Input: part model. Units: mm. Frame: model coordinates. Face numbers are marked on the shaded views. Round coordinates to 2 decimals unless told otherwise and drop trailing zeros. Loops run counter-clockwise (first coordinate to the right, second up) from the corner with the lowest first, then second, coordinate; pieces in that order, holes last.
(1) Cut plane D-D, the plane x = -29. Output: boundary loops of the cut face in (y, z) (3 decimals).
(2) Cut plane B-B, the plane z = 3.5. Output: boundary loops of the cut face in (x, y) (3 decimals).
(3) Line query: line 1 (X direction, y = 67.5, z = 5) (3 decimals); line 2 (Z direction, x = -6.5, y = 2); line 3 (X direction, y = 22.5, z = 1). Output: solid intervals per line, ascending.
(4) Cut plane A-A, the plane y = 81. Output: boundary loops of the cut face in (x, z) (1 decimal).
(5) Draft query along X for the marked faces 1 and 2. Return one class per face: released by +X, released by -X, zero draft, split by the parting line, or undercut.
(6) Cut plane C-C, the plane x = 0. Output: boundary loops of the cut face in (y, z) (1 decimal).
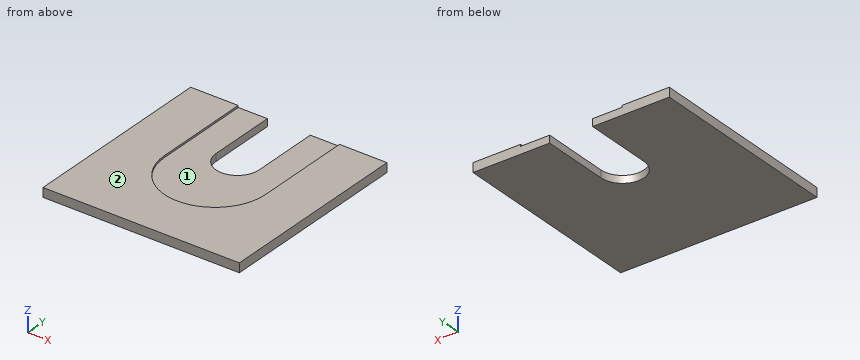
from build123d import *

# Parameters (mm, degrees)
F1_DEPTH = 9.525
F2_DEPTH = 7.62


# Not quite as in the source:
# - a feature names something its author has since deleted; it is built from what else it names


with BuildPart() as f1:
    # F0 (on Top) → F1 (new body)
    with BuildSketch(Plane.XY):
        with BuildLine():
            Line((-101.6, 101.6), (-101.6, -101.6))
            Line((-101.6, -101.6), (101.6, -101.6))
            Line((101.6, -101.6), (101.6, 101.6))
            Line((101.6, 101.6), (52.3875, 101.6))
            Line((52.3875, 101.6), (52.3875, 0))
            ThreePointArc((52.3875, 0), (0, -52.3875), (-52.3875, 0))
            Line((-52.3875, 0), (-52.3875, 101.6))
            Line((-52.3875, 101.6), (-101.6, 101.6))
        make_face()
    extrude(amount=F1_DEPTH)

    # F0 (on Top) → F2 (join)
    with BuildSketch(Plane.XY):
        with BuildLine():
            Line((-22.225, 101.6), (-52.3875, 101.6))
            Line((-52.3875, 101.6), (-52.3875, 0))
            ThreePointArc((-52.3875, 0), (-44.2083835022, 28.1081657953), (-22.225, 47.439430132))
            Line((-22.225, 47.439430132), (-22.225, 101.6))
        make_face()
        with BuildLine():
            Line((52.3875, 0), (52.3875, 101.6))
            Line((52.3875, 101.6), (22.225, 101.6))
            Line((22.225, 101.6), (22.225, 47.439430132))
            ThreePointArc((22.225, 47.439430132), (44.2083835022, 28.1081657953), (52.3875, 0))
        make_face()
        with BuildLine():
            ThreePointArc((-22.225, 47.439430132), (-44.2083835022, 28.1081657953), (-52.3875, 0))
            ThreePointArc((-52.3875, 0), (0, -52.3875), (52.3875, 0))
            ThreePointArc((52.3875, 0), (44.2083835022, 28.1081657953), (22.225, 47.439430132))
            Line((22.225, 47.439430132), (22.225, 31))
            ThreePointArc((22.225, 31), (0, 8.775), (-22.225, 31))
            Line((-22.225, 31), (-22.225, 47.439430132))
        make_face()
    extrude(amount=F2_DEPTH)


solid = f1.part
Reported:
1. outline: (-101.6, 0) - (101.6, 0) - (101.6, 7.62) - (-43.629, 7.62) - (-43.629, 9.525) - (-101.6, 9.525) - close
2. outline: (-101.6, -101.6) - (101.6, -101.6) - (101.6, 101.6) - (22.225, 101.6) - (22.225, 31) arc R22.225 cw to (-22.225, 31) - (-22.225, 101.6) - (-101.6, 101.6) - close
3. line 1: x = -101.6 to -22.225, 22.225 to 101.6
3. line 2: z = 0 to 7.62
3. line 3: x = -101.6 to -20.54, 20.54 to 101.6
4. outline: (-101.6, 0) - (-22.2, 0) - (-22.2, 7.6) - (-52.4, 7.6) - (-52.4, 9.5) - (-101.6, 9.5) - close; (22.2, 0) - (101.6, 0) - (101.6, 9.5) - (52.4, 9.5) - (52.4, 7.6) - (22.2, 7.6) - close
5. face 1: undercut
5. face 2: zero draft
6. outline: (-101.6, 0) - (8.8, 0) - (8.8, 7.6) - (-52.4, 7.6) - (-52.4, 9.5) - (-101.6, 9.5) - close
